from build123d import *

# Parameters (mm, degrees)
SKETCH1_R               = 8.189006913
BOSS_EXTRUDE1_DEPTH     = 20
SKETCH2_R               = 3
CUT_EXTRUDE1_DEPTH      = 30
SKETCH4_W               = 1.839212521
SKETCH4_H               = 4.190652527
BOSS_EXTRUDE2_DEPTH     = 10
SKETCH3_R               = 1.5
CUT_EXTRUDE2_DEPTH      = 10
CUT_EXTRUDE2_DEPTH_BACK = 10


with BuildPart() as part:
    # Sketch1 → Boss-Extrude1 (new body)
    with BuildSketch(Plane(origin=(0, 0, 0), x_dir=(1, 0, 0), z_dir=(0, 1, 0))):
        Circle(SKETCH1_R)
    extrude(amount=BOSS_EXTRUDE1_DEPTH)

    # Sketch2 → Cut-Extrude1 (cut)
    with BuildSketch(Plane(origin=(0, 20, 0), x_dir=(1, 0, 0), z_dir=(0, 1, 0))):
        Circle(SKETCH2_R)
    extrude(amount=-CUT_EXTRUDE1_DEPTH, mode=Mode.SUBTRACT)

    # Sketch4 → Boss-Extrude2 (add)
    with BuildSketch(Plane(origin=(0, 20, 0), x_dir=(1, 0, 0), z_dir=(0, 1, 0))):
        with Locations((-3.214713917, 0.163363311)):
            Rectangle(SKETCH4_W, SKETCH4_H)
    extrude(amount=-BOSS_EXTRUDE2_DEPTH)

    # Sketch3 → Cut-Extrude2 (cut, two sides)
    with BuildSketch(Plane(origin=(0, 0, 0), x_dir=(0, 0, -1), z_dir=(1, 0, 0))) as cut_extrude2_sk:
        with Locations((0, 15)):
            Circle(SKETCH3_R)
    extrude(amount=CUT_EXTRUDE2_DEPTH, mode=Mode.SUBTRACT)
    extrude(cut_extrude2_sk.sketch, amount=-CUT_EXTRUDE2_DEPTH_BACK, mode=Mode.SUBTRACT)


solid = part.part
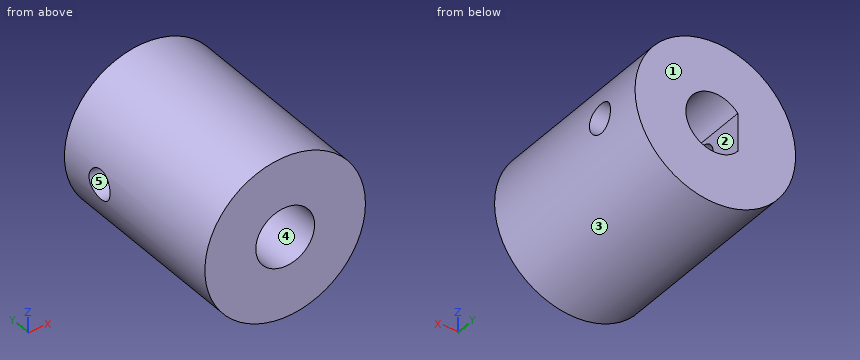
Design review of the part built by this model. Coordinates are the model's own, in mm. Face numbers are marked on the shaded views. A direction names the side the tool comes from. Give positions to 0.01 mm unless a question says otherwise; leave off trailing zeros. Write each loop counter-clockwise with the first axis right and the second up, starting at its lowest first coordinate (ties: lowest second). Pieces come first, ordered by that corner, then holes. Notation, with made-up numbers: M 86.25,-27 L 131.25,-27 A20 ccw 131.25,-7 Z; hole C 2.5,-3 d6. An arc over 180 degrees is marked long. Return JSON: item names as keys, results as strings. Group by question number.
Item 1: Take a section at C-C (y = 15). Give the boundary of the cut face in (x, z), plus the area to 3 significant figures.
Item 2: Take a section at A-A (z = 0). Give the boundary of the cut face in (x, y), plus the area to 3 significant figures.
Item 3: Take a section at D-D (y = 3.75). Give the boundary of the cut face in (x, z).
Item 4: Clearance check with flat-ended pins moving along their axes: pin 1 Ø8 at (y, z) = (5.5, 5.5) entering from -X; pin 2 Ø8 at (y, z) = (18, 5) entering from +X; pin 3 Ø4 at (x, y) = (4, 10) entering from -Z. State where each tip first meets the part, or that it passes through.
Item 5: Tool access review of the marked faces 1 and 2: name each direction out of +Z, -Z, +X, -X, +Y, -Y from which nothing blocks a thin tool from reaching the whole face with its end or side.
Item 6: The part is to be moulded in two halves that separate along X. For the marked faces 3, 4 and 5, say which applies: pulls with the +X half, pulls with the -X half, needs draft (parallel to the pull), parting line crosses it, or undercut.
Item 7: Wall thickness on line 1 along X through (y, z) = (7.5, 0); line 2 along Y through (x, z) = (-4, 0): over which ranges is each line inside the solid? List them lowest first.
Item 8: Take a section at B-B (x = 0). Give the boundary of the cut face in (y, z), plus the area to 3 significant figures.
Return value:
{
 "1": {"outline": "M -8.05,-1.5 A8.19 ccw 8.05,-1.5 L 2.6,-1.5 A3 cw -2.3,-1.93 L -2.3,-1.5 Z; M -8.05,1.5 L -2.3,1.5 L -2.3,1.93 A3 cw 2.6,1.5 L 8.05,1.5 A8.19 ccw Z", "area": "151 mm2"},
 "2": {"outline": "M -8.19,0 L -3,0 L -3,10 L -2.3,10 L -2.3,13.5 L -8.19,13.5 Z; M -8.19,16.5 L -2.3,16.5 L -2.3,20 L -8.19,20 Z; M 3,0 L 8.19,0 L 8.19,13.5 L 3,13.5 Z; M 3,16.5 L 8.19,16.5 L 8.19,20 L 3,20 Z", "area": "181 mm2"},
 "3": {"outline": "C 0,0 d16.38; hole C 0,0 d6"},
 "4": {"pin 1": "stops at x = -8.05", "pin 2": "stops at x = 8.13", "pin 3": "stops at z = -7.94"},
 "5": {"face 1": "+Z, -Z, +X, -X, +Y", "face 2": "+Y, -Y"},
 "6": {"face 3": "parting line crosses it", "face 4": "undercut", "face 5": "needs draft"},
 "7": {"line 1": "x = -8.19 to -3, 3 to 8.19", "line 2": "y = 0 to 13.5, 16.5 to 20"},
 "8": {"outline": "M 0,-8.19 L 20,-8.19 L 20,-3 L 0,-3 Z; M 0,3 L 20,3 L 20,8.19 L 0,8.19 Z", "area": "208 mm2"}
}
